The model under review builds one solid part; all positions refer to its coordinate system, in mm. A direction names the side the tool comes from. Coordinates: 2 decimals unless noted, no trailing zeros. Loops run counter-clockwise (first coordinate to the right, second up) from the corner with the lowest first, then second, coordinate; pieces in that order, holes last. Notation, with made-up numbers: M -34.5,83.5 L 9.5,83.5 A16 cw 9.5,96.5 Z; hole C 26,-30 d5. An arc over 180 degrees is marked long. One line per item, written item: value.
Autodesk Inventor part; units mm, degrees
ref_plane "YZ Plane" through (0, 0, 0) normal (1, 0, 0) x (0, 1, 0)
ref_plane "XZ Plane" through (0, 0, 0) normal (0, 1, 0) x (-1, 0, 0)
ref_plane "XY Plane" through (0, 0, 0) normal (0, 0, 1) x (1, 0, 0)
sketch "Sketch2" plane through (0, 0, 0) normal (0, 0, 1) x (1, 0, 0)
  circle A0 centre (0, 0) radius 22.25
  dimension "d2" = 44.5
extrude "Extrusion1" add sketch "Sketch2" along normal blind 83
sketch "Sketch9" plane through (0, 0, 83) normal (0, 0, 1) x (1, 0, 0)
  circle A0 centre (0, 0) radius 22.25
  line L0 (-31.15, 0) -> (31.15, 0)
  line L1 (0, -31.15) -> (0, 31.15)
  circle A1 centre (0, 0) radius 18
  dimension "d54" = 36
extrude "Extrusion7" cut sketch "Sketch9" against normal blind 81 contours A1 L1 L0 | L0 L1 A1 | L1 L0 A1 | A1 L0 L1
fillet "Fillet12" radius 10 1 edges at (-18, 0, 2)
sketch "Sketch18" plane through (0, 0, 2) normal (0, 0, 1) x (1, 0, 0)
  line L0 (-31.15, 0) -> (31.15, 0)
  line L1 (0, -31.15) -> (0, 31.15)
  line L2 (1.55, 2.35) -> (-1.55, 2.35)
  line L3 (-1.55, 2.35) -> (-1.55, -2.35)
  line L4 (-1.55, -2.35) -> (1.55, -2.35)
  line L5 (1.55, -2.35) -> (1.55, 2.35)
  line L6 (1.55, 2.35) -> (-1.55, -2.35) construction
  line L7 (-1.55, 2.35) -> (1.55, -2.35) construction
  point P0 (0, 0)
  dimension "d122" = 3.1
  dimension "d123" = 4.7
extrude "Extrusion15" cut sketch "Sketch18" against normal through all
chamfer "Chamfer8" distance 2 angle 45 4 edges at (1.55, 0, 2) (0, 2.35, 2) (0, -2.35, 2) (-1.55, 0, 2)
fillet "Fillet13" radius 16 1 edges at (-22.25, 0, 0)
equation "\"BendRadius\" = Thickness"
equation "\"BendReliefWidth\" = Thickness"
equation "\"BendReliefDepth\" = 0.5 * Thickness"
equation "\"CornerReliefSize\" = 4 * Thickness"
equation "\"MinimumRemnant\" = 2 * Thickness"
equation "\"TransitionRadius\" = BendRadius"
equation "\"JacobiRadiusSize\" = BendRadius"
equation "\"GapSize\" = Thickness"
properties part number "_3DPrint"
(1) Add section A-A on z = 69. State the section outline as (x, y) points, then the cut area to 3 significant figures.
Checks:
outline: C 0,0 d44.5; hole C 0,0 d36
area: 537 mm^2
(2) Tool access review of faces 1 (the face through (8.1, -16.4, 83)), 2 (the face through (-2.343, 17.847, 47.997)): name each direction out of +Z, -Z, +X, -X, +Y, -Y from which nothing blocks a thin tool from reaching the whole face with its end or side.
Checks:
face 1: +Z, +X, -X, +Y, -Y
face 2: +Z
(3) To check wall thickness, follow L1, parallel to Y at x = 0, z = 48; L2, parallel to X at y = 14, z = 7; L3, parallel to X at y = -10.5, z = 28.5. State the ranges of each line that lie inside material, in increasing order. Write a range as [from, to].
Checks:
L1: [-22.25, -18], [18, 22.25]
L2: [-13.54, -9.03], [9.03, 13.54]
L3: [-19.62, -14.62], [14.62, 19.62]
(4) Draft analysis for pull direction X (two halves, no side actions). For faces 3 (the face through (-16.399, -15.038, 49.031)), 4 (the face through (0, -3, 0)), 5 (the face through (-4, 0, 2)), state which applies: pulls with the +X half, pulls with the -X half, needs draft (parallel to the pull), parting line crosses it, or undercut.
Checks:
face 3: parting line crosses it
face 4: needs draft
face 5: undercut
(5) Insertion check: pin 1 Ø1 at (x, y) = (-2.5, -7) entering from +Z; pin 2 Ø8 at (y, z) = (-16, 49.5) entering from +X; pin 3 Ø4 at (y, z) = (-17.5, 66.5) entering from -X. Each pin has a flat end and moves straight along its axis. Give the tip position at first contact, or say it passes through.
Checks:
pin 1: z = 2
pin 2: x = 18.74
pin 3: x = -15.96
